```python
from build123d import *

# Parameters (mm, degrees)
F0_W     = 25
F0_H     = 25
F1_DEPTH = 25
F2_R     = 3.125
F3_DEPTH = 25.4
F4_R     = 3.125
F5_DEPTH = 25.4
F6_R     = 3.125
F7_DEPTH = 25.4
F8_R     = 5.08
F9_R     = 5.08
F10_R    = 5.08
F11_R    = 5.08
F12_R    = 5.08
F13_R    = 5.08


with BuildPart() as f1:
    # F0 (on Top) → F1 (new body)
    with BuildSketch(Plane.XY):
        with Locations((12.5, -12.5)):
            Rectangle(F0_W, F0_H)
    extrude(amount=F1_DEPTH)

    # F2 (on face) → F3 (cut)
    with BuildSketch(Plane.XZ.offset(25)):
        with Locations((12.5, 12.5)):
            Circle(F2_R)
    extrude(amount=-F3_DEPTH, mode=Mode.SUBTRACT)

    # F4 (on face) → F5 (cut)
    with BuildSketch(Plane.YZ.offset(25)):
        with Locations((-12.5, 12.5)):
            Circle(F4_R)
    extrude(amount=-F5_DEPTH, mode=Mode.SUBTRACT)

    # F6 (on face) → F7 (cut)
    with BuildSketch(Plane.XY.offset(25)):
        with Locations((12.5, -12.5)):
            Circle(F6_R)
    extrude(amount=-F7_DEPTH, mode=Mode.SUBTRACT)

    # F8
    f8_edges = [f1.edges().sort_by_distance(p)[0] for p in [
        (12.5, -25, 0),
    ]]
    fillet(f8_edges, radius=F8_R)

    # F9
    f9_edges = [f1.edges().sort_by_distance(p)[0] for p in [
        (12.5, 0, 0),
    ]]
    fillet(f9_edges, radius=F9_R)

    # F10
    f10_edges = [f1.edges().sort_by_distance(p)[0] for p in [
        (12.5, 0, 25),
    ]]
    fillet(f10_edges, radius=F10_R)

    # F11
    f11_edges = [f1.edges().sort_by_distance(p)[0] for p in [
        (12.5, -25, 25),
    ]]
    fillet(f11_edges, radius=F11_R)

    # F12
    f12_edges = [f1.edges().sort_by_distance(p)[0] for p in [
        (25, 0, 12.5),
    ]]
    fillet(f12_edges, radius=F12_R)

    # F13
    f13_edges = [f1.edges().sort_by_distance(p)[0] for p in [
        (0, -12.5, 25),
    ]]
    fillet(f13_edges, radius=F13_R)


solid = f1.part
```
Part model, mm, in its own coordinate system. Give positions to 0.01 mm unless a question says otherwise; leave off trailing zeros. Write each loop counter-clockwise with the first axis right and the second up, starting at its lowest first coordinate (ties: lowest second). Pieces come first, ordered by that corner, then holes. Notation, with made-up numbers: (-2, 65.25) -> (49, 65.25) arc R19 ccw to (49, 89.25) -> close; hole circle Ø1 at (-23.5, -19.5). An arc over 180 degrees is marked (long way). Put each result on its own line as item: value. Start each with the question number.
Item 1: Pin check, flat tip, straight feed: pin 1 Ø4 at (x, y) = (17.5, -2.5) entering from -Z. Stop position of the tip, or through.
Item 2: Cut at A-A (z = 12.5). List the corners of the cut face in (x, y) (3 decimals), then the cut area to 3 significant figures.
Item 3: Cut at B-B (y = -12.5). List the corners of the cut face in (x, z) (3 decimals), then the cut area to 3 significant figures.
Item 4: Cut at C-C (x = 4.5). List the corners of the cut face in (y, z) (3 decimals), then the cut area to 3 significant figures.
Item 5: Pull direction Z, two halves, no side cores. Call faces 1 (the face through (9.38, -19.93, 12.64)), 2 (the face through (23.472, -12.604, 23.551)), 3 (the face through (1.528, -23.551, 12.604)): pulls with the +Z half, pulls with the -Z half, needs draft (parallel to the pull), parting line crosses it, or undercut.
Item 6: Wall check: L1, parallel to X at y = -16, z = 12.5 (3 decimals); L2, parallel to Y at x = 20.25, z = 12.75; L3, parallel to Y at x = 1.5, z = 9.75. Give the ranges that are in metal, low to high. Write a range as [from, to].
Item 7: Cut at D-D (z = 8.5). List the corners of the cut face in (x, y) (3 decimals), then the cut area to 3 significant figures.
Answer list:
1. pin 1: stops at z = 0.03
2. outline: (0, -19.92) arc R5.08 ccw to (5.08, -25) -> (9.375, -25) -> (9.375, -15.625) -> (0, -15.625) -> close; (0, -9.375) -> (9.375, -9.375) -> (9.375, 0) -> (5.08, 0) arc R5.08 ccw to (0, -5.08) -> close; (15.625, -25) -> (19.92, -25) arc R5.08 ccw to (25, -19.92) -> (25, -15.625) -> (15.625, -15.625) -> close; (15.625, -9.375) -> (25, -9.375) -> (25, -5.08) arc R5.08 ccw to (19.92, 0) -> (15.625, 0) -> close
2. area: 329 mm2
3. outline: (0, 5.08) arc R5.08 ccw to (5.08, 0) -> (9.375, 0) -> (9.375, 9.375) -> (0, 9.375) -> close; (0, 15.625) -> (9.375, 15.625) -> (9.375, 25) -> (5.08, 25) arc R5.08 ccw to (0, 19.92) -> close; (15.625, 0) -> (19.92, 0) arc R5.08 ccw to (25, 5.08) -> (25, 9.375) -> (15.625, 9.375) -> close; (15.625, 15.625) -> (25, 15.625) -> (25, 19.92) arc R5.08 ccw to (19.92, 25) -> (15.625, 25) -> close
3. area: 329 mm2
4. outline: (-24.967, 5.08) arc R5.047 ccw to (-19.92, 0.033) -> (-5.08, 0.033) arc R5.047 ccw to (-0.033, 5.08) -> (-0.033, 19.92) arc R5.047 ccw to (-5.08, 24.967) -> (-19.92, 24.967) arc R5.047 ccw to (-24.967, 19.92) -> close; hole circle Ø6.25 at (-12.5, 12.5)
4. area: 569 mm2
5. face 1: undercut
5. face 2: pulls with the +Z half
5. face 3: needs draft
6. L1: x = [0, 9.375], [15.625, 25]
6. L2: y = [-24.99, -15.61], [-9.39, -0.01]
6. L3: y = [-23.52, -13.98], [-11.02, -1.48]
7. outline: (0, -19.92) arc R5.08 ccw to (5.08, -25) -> (19.92, -25) arc R5.08 ccw to (25, -19.92) -> (25, -5.08) arc R5.08 ccw to (19.92, 0) -> (5.08, 0) arc R5.08 ccw to (0, -5.08) -> close; hole circle Ø6.25 at (12.5, -12.5)
7. area: 572 mm2
